from build123d import *

# Parameters (mm, degrees)
F4_DEPTH = 3.175
F3_R     = 1.5
F5_DEPTH = 3.175


with BuildPart() as f4:
    # F2 (on face) → F4 (new body)
    with BuildSketch(Plane.XY):
        Polygon((-14.01338, -42.228443), (-223.278188, 78.114037), (-223.278188, -161.413451), (-170.104977, -161.413451), align=None)
    extrude(amount=F4_DEPTH)

    # F3 (on Top) → F5 (cut)
    with BuildSketch(Plane.XY):
        with Locations((-160.294694, -144.486368)):
            Circle(F3_R)
        with Locations((-124.965932, -117.510804)):
            Circle(F3_R)
        with Locations((-89.637169, -90.53524)):
            Circle(F3_R)
        with Locations((-54.308407, -63.559676)):
            Circle(F3_R)
        with Locations((-54.308407, -27.707599)):
            Circle(F3_R)
        with Locations((-87.336499, -8.714044)):
            Circle(F3_R)
        with Locations((-120.364591, 10.27951)):
            Circle(F3_R)
        with Locations((-153.392684, 29.273065)):
            Circle(F3_R)
        with Locations((-215.778188, -143.52337)):
            Circle(F3_R)
        with Locations((-215.778188, -105.42337)):
            Circle(F3_R)
        with Locations((-215.778188, -67.32337)):
            Circle(F3_R)
        with Locations((-215.778188, -29.22337)):
            Circle(F3_R)
        with Locations((-215.778188, 46.97663)):
            Circle(F3_R)
        with Locations((-186.420776, 48.26662)):
            Circle(F3_R)
        with Locations((-215.778188, 8.87663)):
            Circle(F3_R)
    extrude(amount=F5_DEPTH, mode=Mode.SUBTRACT)


solid = f4.part
For this review, take the finished solid that the model builds, in its own axes (mm). Round coordinates to 2 decimals unless told otherwise and drop trailing zeros. Write each loop counter-clockwise with the first axis right and the second up, starting at its lowest first coordinate (ties: lowest second). Pieces come first, ordered by that corner, then holes. Notation, with made-up numbers: M 36.5,77.5 L 42.5,77.5 A25 ccw 42.5,112.5 Z; hole C 31.25,-30 d5. An arc over 180 degrees is marked long. Write item = value, one per line. Start each with the question number.
(1) Clearance check with flat-ended pins moving along their axes: pin 1 Ø4 at (x, y) = (-215.78, -67.32) entering from +Z (3 decimals); pin 2 Ø1 at (x, z) = (-115, 1) entering from -Y; pin 3 Ø1.5 at (x, z) = (-119.5, 1) entering from -Y. State where each tip first meets the part, or that it passes through.
(2) We need section B-B (x = -199). Give the boundary of the cut face in (y, z) (3 decimals).
(3) We need section C-C (y = -16). Give the boundary of the cut face in (x, z) (3 decimals).
(4) For line 1 along X through (y, z) = (-116.5, 0.5); line 2 along Y through (x, z) = (-161, 0.35); line 3 along Y through (x, z) = (-86.5, 0.7), list the stretches that pass through material, from the lowest coordinate up.
(5) We need section A-A (z = 1.3). Give the number of separate pieces and of enclosed holes in the cut face, then the cut area to 3 significant figures.
Results found:
q1.pin_1 = 3.175
q1.pin_2 = -119.72
q1.pin_3 = -123.35
q2.outline = M -161.413,0 L 64.152,0 L 64.152,3.175 L -161.413,3.175 Z
q3.outline = M -223.278,0 L -59.622,0 L -59.622,3.175 L -223.278,3.175 Z
q4.line_1 = -223.28 to -126.07, -123.86 to -111.28
q4.line_2 = -154.46 to -145.81, -143.16 to 42.3
q4.line_3 = -97.58 to -9.96, -7.47 to -0.54
q5.separate_pieces = 1
q5.enclosed_holes = 15
q5.area = 28,100 mm²
